Autodesk Fusion 360 part; units mm, degrees
sketch "Sketch1" plane through (0, 0, 0) normal (0, 0, 1) x (1, 0, 0)
  line L0 (0, 0) -> (175, 0)
  line L1 (175, 0) -> (175, 140)
  line L2 (175, 140) -> (0, 140)
  line L3 (0, 140) -> (0, 0)
  line L4 (50, 140) -> (50, 0)
  line L5 (125, 140) -> (125, 0)
  circle A0 centre (57.5, 5) radius 1.35
  circle A1 centre (117.5, 5) radius 1.35
  line L6 (87.5, 0) -> (87.5, 140) construction
  circle A2 centre (57.5, 135) radius 1.35
  circle A3 centre (117.5, 135) radius 1.35
  dimension "d1" = 140
  dimension "d2" = 175
  dimension "d3" = 50
  dimension "d4" = 50
  dimension "d5" = 2.7
  dimension "d6" = 5
  dimension "d7" = 2.7
  dimension "d8" = 5
  dimension "d10" = 60
  dimension "d11" = 2.7
  dimension "d12" = 2.7
  dimension "d13" = 60
  dimension "d14" = 5
  dimension "d15" = 5
extrude "Extrude1" add sketch "Sketch1" along normal blind 20 contours L0 L2 L4 L5
extrude "Extrude2" add sketch "Sketch1" along normal blind 15 contours A0 | A1 | A2 | A3
extrude "Extrude3" add sketch "Sketch1" along normal blind 5 contours L0 L2 L3 L4 | L0 L1 L2 L5
Source: CAD feature listing. Evaluate the final solid. Frame: model axes, mm. A direction names the side the tool comes from. Coordinates: 2 decimals unless noted, no trailing zeros. Order: outer loops, then holes, each group sorted by start corner. A loop starts at its lowest first (then second) coordinate and runs counter-clockwise, first axis right, second up. Notation, with made-up numbers: M 88.25,84 L 127.25,84 A24 ccw 127.25,107 Z; hole C 41,81 d6. An arc over 180 degrees is marked long. Write each question's results on one line, items separated by ' | '. Start each with the question number.
1. Section B-B, the plane z = 12.5. Return the cut outline in (x, y).
2. Pin query (flat end, axial travel): pin 1 (2 mm diameter, centred on x = 117.5, y = 135, fed in from +Z); pin 2 (2 mm diameter, centred on y = 24.5, z = 17, fed in from -X); pin 3 (2 mm diameter, centred on y = 80, z = 16.5, fed in from +X). Return the tip coordinate at first contact, or that it passes through.
3. Material intervals for L1, parallel to Y at x = 117.5, z = 16.85; L2, parallel to X at y = 135, z = 18.1; L3, parallel to X at y = 133, z = 19, sorted ascending.
4. Reachability of faces 1 (the face through (150, 71, 5)), 2 (the face through (86, 71, 0)), 3 (the face through (50, 71, 12)) from +Z, -Z, +X, -X, +Y, -Y: full face, straight path, thin tool, end or side. Return the list, or none.
5. Section C-C, the plane x = 142. Return the cut outline in (y, z).
6. Section A-A, the plane y = 64. Return the cut outline in (x, z), then the cut area to 3 significant figures.
Solution:
1) outline: M 50,0 L 125,0 L 125,140 L 50,140 Z
2) pin 1: z = 15 | pin 2: x = 50 | pin 3: x = 125
3) L1: 0 to 3.65, 6.35 to 133.65, 136.35 to 140 | L2: 50 to 56.15, 58.85 to 116.15, 118.85 to 125 | L3: 50 to 125
4) face 1: +Z, +X, +Y, -Y | face 2: -Z, +X, -X, +Y, -Y | face 3: +Z, -X, +Y, -Y
5) outline: M 0,0 L 140,0 L 140,5 L 0,5 Z
6) outline: M 0,0 L 175,0 L 175,5 L 125,5 L 125,20 L 50,20 L 50,5 L 0,5 Z | area: 2,000 mm²
